```python
from build123d import *

# Parameters (mm, degrees)
F0_W         = 27
F0_H         = 27
F1_DEPTH     = 0.6
F2_DEPTH     = 6
F3_R         = 2
F4_T1_DEPTH  = 5.4
F4_T4_ANGLE  = 90
F4_T6_ANGLE  = 90
F4_T8_ANGLE  = 90
F4_T10_ANGLE = 90
F5_W         = 5
F5_H         = 2.8
F6_DEPTH     = 5.6
F7_W         = 6
F7_H         = 3
F8_DEPTH     = 6
F9_R         = 2
F10_DEPTH    = 4


# Not quite as in the source:
# - a fillet or chamfer that OpenCascade refuses, or shapes differently, is made with other operations: its cross-section is extruded or revolved along the edge and cut away or added


with BuildPart() as f1:
    # F0 (on Top) → F1 (new body)
    with BuildSketch(Plane.XY):
        with BuildLine():
            Line((-40.6, 95), (-60.6, 80))
            Line((-60.6, 80), (-60.6, 0))
            Line((-60.6, 0), (60.6, 0))
            Line((60.6, 0), (60.6, 80))
            Line((60.6, 80), (40.6, 95))
            Line((40.6, 95), (20.6, 146.2347538298))
            ThreePointArc((20.6, 146.2347538298), (0, 160.3072328817), (-20.6, 146.2347538298))
            Line((-20.6, 146.2347538298), (-40.6, 95))
        make_face()
        with Locations((0, 118.5)):
            Rectangle(F0_W, F0_H, mode=Mode.SUBTRACT)
        with Locations((0, 118.5)):
            Rectangle(F0_W, F0_H)
    extrude(amount=F1_DEPTH)

    # F0 (on Top) → F2 (join)
    with BuildSketch(Plane.XY):
        with Locations((0, 118.5)):
            Rectangle(F0_W, F0_H)
    extrude(amount=F2_DEPTH)

    # F3
    f3_edges = [f1.edges().sort_by_distance(p)[0] for p in [
        (0, 132, 6),
        (-13.5, 118.5, 6),
        (0, 105, 6),
        (13.5, 118.5, 6),
    ]]
    fillet(f3_edges, radius=F3_R)

    # F4: fillet of radius 3 on 4 edges, made by hand

    # F4_s2 → F4_t1 (cut)
    with BuildSketch(Plane.XY.offset(0.6)):
        with BuildLine():
            ThreePointArc((-13.5, 129), (-12.6213203436, 131.1213203436), (-10.5, 132))
            Line((-10.5, 132), (-13.5, 132))
            Line((-13.5, 132), (-13.5, 129))
        make_face()
        with BuildLine():
            ThreePointArc((-13.5, 108), (-12.6213203436, 105.8786796564), (-10.5, 105))
            Line((-10.5, 105), (-13.5, 105))
            Line((-13.5, 105), (-13.5, 108))
        make_face()
        with BuildLine():
            ThreePointArc((10.5, 105), (12.6213203436, 105.8786796564), (13.5, 108))
            Line((13.5, 108), (13.5, 105))
            Line((13.5, 105), (10.5, 105))
        make_face()
        with BuildLine():
            ThreePointArc((10.5, 132), (12.6213203436, 131.1213203436), (13.5, 129))
            Line((13.5, 129), (13.5, 132))
            Line((13.5, 132), (10.5, 132))
        make_face()
    extrude(amount=F4_T1_DEPTH, mode=Mode.SUBTRACT)

    # F4_s3 → F4_t4 (revolve, cut)
    with BuildSketch(Plane.XZ.offset(-129)):
        with BuildLine():
            ThreePointArc((11.5, 6), (12.9142135624, 5.4142135624), (13.5, 4))
            Line((13.5, 4), (13.5, 6))
            Line((13.5, 6), (11.5, 6))
        make_face()
    revolve(axis=Axis((10.5, 129, 6), (0, 0, 1)), revolution_arc=F4_T4_ANGLE, mode=Mode.SUBTRACT)

    # F4_s5 → F4_t6 (revolve, cut)
    with BuildSketch(Plane.YZ.offset(10.5)):
        with BuildLine():
            ThreePointArc((107, 6), (105.5857864376, 5.4142135624), (105, 4))
            Line((105, 4), (105, 6))
            Line((105, 6), (107, 6))
        make_face()
    revolve(axis=Axis((10.5, 108, 6), (0, 0, 1)), revolution_arc=F4_T6_ANGLE, mode=Mode.SUBTRACT)

    # F4_s7 → F4_t8 (revolve, cut)
    with BuildSketch(Plane.XZ.offset(-108)):
        with BuildLine():
            ThreePointArc((-11.5, 6), (-12.9142135624, 5.4142135624), (-13.5, 4))
            Line((-13.5, 4), (-13.5, 6))
            Line((-13.5, 6), (-11.5, 6))
        make_face()
    revolve(axis=Axis((-10.5, 108, 6), (0, 0, 1)), revolution_arc=F4_T8_ANGLE, mode=Mode.SUBTRACT)

    # F4_s9 → F4_t10 (revolve, cut)
    with BuildSketch(Plane.YZ.offset(-10.5)):
        with BuildLine():
            ThreePointArc((130, 6), (131.4142135624, 5.4142135624), (132, 4))
            Line((132, 4), (132, 6))
            Line((132, 6), (130, 6))
        make_face()
    revolve(axis=Axis((-10.5, 129, 6), (0, 0, 1)), revolution_arc=F4_T10_ANGLE, mode=Mode.SUBTRACT)

    # F5 (on face) → F6 (join)
    with BuildSketch(Plane.XY.offset(0.6)):
        with Locations((-58.1, 70.5)):
            Rectangle(F5_W, F5_H)
        with Locations((-58.1, 64.5)):
            Rectangle(F5_W, F5_H)
        with Locations((58.1, 70.5)):
            Rectangle(F5_W, F5_H)
        with Locations((58.1, 64.5)):
            Rectangle(F5_W, F5_H)
    extrude(amount=F6_DEPTH)

    # F7 (on face) → F8 (join)
    with BuildSketch(Plane.XY.offset(0.6)):
        with Locations((-56.6, 1.5)):
            Rectangle(F7_W, F7_H)
        with Locations((56.6, 1.5)):
            Rectangle(F7_W, F7_H)
        with Locations((0, 1.5)):
            Rectangle(F7_W, F7_H)
    extrude(amount=F8_DEPTH)

    # F9 (on face) → F10 (cut)
    with BuildSketch(Plane.XZ):
        with Locations((56.6, 3.6)):
            Circle(F9_R)
        with Locations((-56.6, 3.6)):
            Circle(F9_R)
        with Locations((0, 3.6)):
            Circle(F9_R)
    extrude(amount=-F10_DEPTH, mode=Mode.SUBTRACT)


solid = f1.part
```
Read the model definition and answer for the solid it produces. Units are mm, in the model's axes. A direction names the side the tool comes from. Round coordinates to 2 decimals unless told otherwise and drop trailing zeros. Write each loop counter-clockwise with the first axis right and the second up, starting at its lowest first coordinate (ties: lowest second). Pieces come first, ordered by that corner, then holes. Notation, with made-up numbers: (3, -2.5) -> (49, -2.5) arc R24 cw to (49, 24.5) -> close; hole circle Ø1 at (39.5, -39). An arc over 180 degrees is marked (long way). Answer in a Markdown table with one row per item. Add a question column.
1) Which of the six approach directions +Z, -Z, +X, -X, +Y, -Y give full straight-line access (tool end or side, diameter ignored) to faces 1 (the face through (-0.434, 1.479, 1.648)), 2 (the face through (-30.46, 120.98, 0.3)), 3 (the face through (-1, 63, 0)), 4 (the face through (13.5, 118, 2)), 5 (the face through (0, 105, 2))?
2) Determine the mould class of faces 6 (the face through (-59, 3, 4)), 7 (the face through (-60.6, 49.1, 0.3)), 8 (the face through (58, 71.9, 3)) for opening direction Y: pulls with the +Y half, pulls with the -Y half, needs draft (parallel to the pull), parting line crosses it, or undercut.
3) Find section C-C, the plane x = -18. Determine the outline of the cut face in (y, z), and give its area (3 significant figures).
4) Consider line 1 (Z direction, x = 0, y = 1.8); line 2 (Z direction, x = 18, y = 39); line 3 (Z direction, x = 56, y = 1). Determine where each line is inside the solid, lowest interval first.
5) Find section A-A, the plane x = 0. Determine the outline of the cut face in (y, z).
6) Find section B-B, the plane y = 151. Determine the outline of the cut face in (x, z).
7) Given P1, Ø2, axis at x = -14.5, y = 34, coming from the +Z side; P2, Ø1.5, axis at x = 57, z = 4.5, coming from the +Y side; P3, Ø2, axis at x = 58, y = 65, coming from the +Z side, each flat-ended and moving along its own axis, determine where each tip first touches the part or whether it passes through.
Findings below:
| question | item | result |
|---|---|---|
| 1 | face 1 | -Y |
| 1 | face 2 | +Z, -Z, -X, +Y |
| 1 | face 3 | -Z, +X, -X, +Y, -Y |
| 1 | face 4 | +Z, +X, +Y, -Y |
| 1 | face 5 | +Z, +X, -X |
| 2 | face 6 | undercut |
| 2 | face 7 | needs draft |
| 2 | face 8 | pulls with the +Y half |
| 3 | outline | (0, 0) -> (151.04, 0) -> (151.04, 0.6) -> (0, 0.6) -> close |
| 3 | area | 90.6 mm² |
| 4 | line 1 | 0 to 1.6, 5.6 to 6.6 |
| 4 | line 2 | 0 to 0.6 |
| 4 | line 3 | 0 to 1.69, 5.51 to 6.6 |
| 5 | outline | (0, 0) -> (160.31, 0) -> (160.31, 0.6) -> (132, 0.6) -> (132, 4) arc R2 ccw to (130, 6) -> (107, 6) arc R2 ccw to (105, 4) -> (105, 0.6) -> (3, 0.6) -> (3, 1.6) -> (0, 1.6) -> close; (0, 5.6) -> (3, 5.6) -> (3, 6.6) -> (0, 6.6) -> close |
| 6 | outline | (-18.03, 0) -> (18.03, 0) -> (18.03, 0.6) -> (-18.03, 0.6) -> close |
| 7 | P1 | z = 0.6 |
| 7 | P2 | y = 71.9 |
| 7 | P3 | z = 6.2 |
